For this review, take the finished solid that the model builds, in its own axes (mm). Face numbers are marked on the shaded views. Coordinates: 2 decimals unless noted, no trailing zeros. Loops run counter-clockwise (first coordinate to the right, second up) from the corner with the lowest first, then second, coordinate; pieces in that order, holes last.
1. Mouldability with a two-part tool opening along X and no side actions: class the marked faces 1, 2 and 3 as pulls with the +X half, pulls with the -X half, needs draft (parallel to the pull), parting line crosses it, or undercut.
2. Clearance check with flat-ended pins moving along their axes: P1, Ø1.6, axis at y = 68, z = 5, coming from the -X side; P2, Ø2.5, axis at x = 23.5, z = 6, coming from the +Y side; P3, Ø2, axis at x = -28, y = 48, coming from the +Z side; P4, Ø3, axis at y = 20, z = 5, coming from the +X side. State where each tip first meets the part, or that it passes through.
3. Take a section at A-A, the plane y = 36.5. State the section outline as (x, z) points.
4. Take a section at B-B, the plane x = 52. State the section outline as (y, z) points.
5. To check wall thickness, follow probe 1 along Y at (x, z) = (-57.5, 5); probe 2 along Z at (x, y) = (57.15, 68); probe 3 along X at (y, z) = (67, 1). State the ranges of each line that lie inside material, in increasing order.
6. Take a section at C-C, the plane z = 2. State the section outline as (x, y) points.
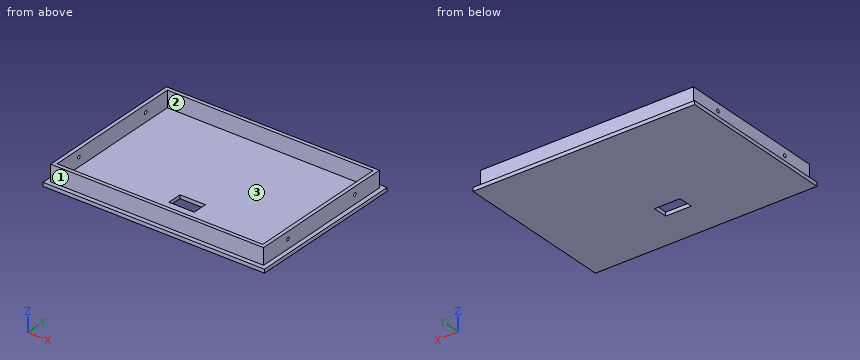
```python
from build123d import *

# Parameters (mm, degrees)
BOSS_EXTRUDE1_START = -2
SKETCH1_W           = 122
SKETCH1_H           = 88
BOSS_EXTRUDE1_DEPTH = 2
BOSS_EXTRUDE2_START = -0.5
SKETCH2_W           = 117.2
SKETCH2_H           = 83.2
BOSS_EXTRUDE2_DEPTH = 9.5
SKETCH3_W           = 113.2
SKETCH3_H           = 79.2
BOSS_EXTRUDE3_DEPTH = 10
BOSS_EXTRUDE4_START = -3
SKETCH4_W           = 14
SKETCH4_H           = 8
BOSS_EXTRUDE4_DEPTH = 4
BOSS_EXTRUDE5_START = -65
SKETCH5_R           = 0.9
BOSS_EXTRUDE5_DEPTH = 130
BOSS_EXTRUDE6_START = -65
SKETCH6_R           = 0.9
BOSS_EXTRUDE6_DEPTH = 130


with BuildPart() as part:
    # Sketch1 → Boss-Extrude1 (new body)
    with BuildSketch(Plane.XY.offset(BOSS_EXTRUDE1_START)):
        with Locations((0, 44)):
            Rectangle(SKETCH1_W, SKETCH1_H)
    extrude(amount=BOSS_EXTRUDE1_DEPTH)

    # Sketch2 → Boss-Extrude2 (add)
    with BuildSketch(Plane.XY.offset(BOSS_EXTRUDE2_START)):
        with Locations((0, 44)):
            Rectangle(SKETCH2_W, SKETCH2_H)
    extrude(amount=BOSS_EXTRUDE2_DEPTH)


with BuildPart() as body_2:
    # Sketch3 → Boss-Extrude3 (new body)
    with BuildSketch(Plane.XY):
        with Locations((0, 44)):
            Rectangle(SKETCH3_W, SKETCH3_H)
    extrude(amount=BOSS_EXTRUDE3_DEPTH)


with BuildPart() as part_1:
    add(part.part)

    # Combine1: cut body 2
    add(body_2.part, mode=Mode.SUBTRACT)


with BuildPart() as body_2_2:
    # Sketch4 → Boss-Extrude4 (new body)
    with BuildSketch(Plane.XY.offset(BOSS_EXTRUDE4_START)):
        with Locations((0, 24)):
            Rectangle(SKETCH4_W, SKETCH4_H)
    extrude(amount=BOSS_EXTRUDE4_DEPTH)


with BuildPart() as part_2:
    add(part_1.part)

    # Combine2: cut body 2 2
    add(body_2_2.part, mode=Mode.SUBTRACT)


with BuildPart() as body_2_3:
    # Sketch5 → Boss-Extrude5 (new body)
    with BuildSketch(Plane(origin=(0, 0, 0), x_dir=(0, 0, -1), z_dir=(1, 0, 0)).offset(BOSS_EXTRUDE5_START)):
        with Locations((-5, 20)):
            Circle(SKETCH5_R)
    extrude(amount=BOSS_EXTRUDE5_DEPTH)


with BuildPart() as part_3:
    add(part_2.part)

    # Combine3: cut body 2 3
    add(body_2_3.part, mode=Mode.SUBTRACT)


with BuildPart() as body_2_4:
    # Sketch6 → Boss-Extrude6 (new body)
    with BuildSketch(Plane(origin=(0, 0, 0), x_dir=(0, 0, -1), z_dir=(1, 0, 0)).offset(BOSS_EXTRUDE6_START)):
        with Locations((-5, 68)):
            Circle(SKETCH6_R)
    extrude(amount=BOSS_EXTRUDE6_DEPTH)


with BuildPart() as part_4:
    add(part_3.part)

    # Combine4: cut body 2 4
    add(body_2_4.part, mode=Mode.SUBTRACT)


solid = part_4.part
```
Results list:
1. face 1: needs draft
1. face 2: undercut
1. face 3: undercut
2. P1: passes through
2. P2: stops at y = 85.6
2. P3: stops at z = 0
2. P4: stops at x = 58.6
3. outline: (-61, -2) - (61, -2) - (61, 0) - (58.6, 0) - (58.6, 9) - (56.6, 9) - (56.6, 0) - (-56.6, 0) - (-56.6, 9) - (-58.6, 9) - (-58.6, 0) - (-61, 0) - close
4. outline: (0, -2) - (88, -2) - (88, 0) - (85.6, 0) - (85.6, 9) - (83.6, 9) - (83.6, 0) - (4.4, 0) - (4.4, 9) - (2.4, 9) - (2.4, 0) - (0, 0) - close
5. probe 1: y = 2.4 to 19.1, 20.9 to 67.1, 68.9 to 85.6
5. probe 2: z = -2 to 4.1, 5.9 to 9
5. probe 3: x = -58.6 to -56.6, 56.6 to 58.6
6. outline: (-58.6, 2.4) - (58.6, 2.4) - (58.6, 85.6) - (-58.6, 85.6) - close; hole (-56.6, 4.4) - (56.6, 4.4) - (56.6, 83.6) - (-56.6, 83.6) - close
